Here's how the part is built. I have some questions about the finished solid (model axes, mm). A direction names the side the tool comes from. Round coordinates to 2 decimals unless told otherwise and drop trailing zeros. Loops run counter-clockwise (first coordinate to the right, second up) from the corner with the lowest first, then second, coordinate; pieces in that order, holes last. Notation, with made-up numbers: M 73,-15.5 L 107,-15.5 A25 ccw 107,10.5 Z; hole C -14,-2 d4. An arc over 180 degrees is marked long. Answer as CSV lines item,"result".
```python
from build123d import *

# Parameters (mm, degrees)
SKETCH1_R           = 6
SKETCH1_R_2         = 15
BOSS_EXTRUDE1_DEPTH = 5


with BuildPart() as part:
    # Sketch1 → Boss-Extrude1 (new body)
    with BuildSketch(Plane(origin=(0, 0, 0), x_dir=(1, 0, 0), z_dir=(0, 1, 0))):
        with BuildLine():
            Line((0, 0), (155, 0))
            Line((155, 0), (155, 20))
            ThreePointArc((155, 20), (152.071067812, 27.071067812), (145, 30))
            Line((145, 30), (119.160797831, 30))
            ThreePointArc((119.160797831, 30), (112.705825587, 32.362373842), (109.300664859, 38.333333333))
            ThreePointArc((109.300664859, 38.333333333), (95.355339059, 65.355339059), (68.333333333, 79.300664859))
            ThreePointArc((68.333333333, 79.300664859), (62.362373842, 82.705825587), (60, 89.160797831))
            Line((60, 89.160797831), (60, 100))
            ThreePointArc((60, 100), (57.071067812, 107.071067812), (50, 110))
            Line((50, 110), (10, 110))
            ThreePointArc((10, 110), (2.928932188, 107.071067812), (0, 100))
            Line((0, 100), (0, 0))
        make_face()
        with Locations((20, 15)):
            Circle(SKETCH1_R, mode=Mode.SUBTRACT)
        with Locations((40, 15)):
            Circle(SKETCH1_R, mode=Mode.SUBTRACT)
        with Locations((60, 15)):
            Circle(SKETCH1_R, mode=Mode.SUBTRACT)
        with Locations((80, 15)):
            Circle(SKETCH1_R, mode=Mode.SUBTRACT)
        with Locations((100, 15)):
            Circle(SKETCH1_R, mode=Mode.SUBTRACT)
        with Locations((120, 15)):
            Circle(SKETCH1_R, mode=Mode.SUBTRACT)
        with Locations((140, 15)):
            Circle(SKETCH1_R, mode=Mode.SUBTRACT)
        with Locations((30, 90)):
            Circle(SKETCH1_R_2, mode=Mode.SUBTRACT)
        with BuildLine():
            Line((60, 60), (30, 60))
            ThreePointArc((30, 60), (22.928932188, 57.071067812), (20, 50))
            Line((20, 50), (20, 40))
            ThreePointArc((20, 40), (22.928932188, 32.928932188), (30, 30))
            Line((30, 30), (77.320508076, 30))
            ThreePointArc((77.320508076, 30), (85.980762114, 35), (85.980762114, 45))
            ThreePointArc((85.980762114, 45), (75, 55.980762114), (60, 60))
        make_face(mode=Mode.SUBTRACT)
    extrude(amount=BOSS_EXTRUDE1_DEPTH)


solid = part.part
```
1. We'd pull the mould along X, two halves only. Please class faces 1 (the cylindrical face through (112.78, 2.46, -32.3)), 2 (the flat face through (76, 0, -56)), 3 (the cylindrical face through (22.85, 2.46, -33.01)): pulls with the +X half, pulls with the -X half, needs draft (parallel to the pull), parting line crosses it, or undercut.
Evaluation:
face 1,"pulls with the +X half"
face 2,"needs draft"
face 3,"undercut"
2. I want a section at A-A, the plane z = -15. Count the separate pieces of the cut face and the enclosed holes in it, and give its area (3 significant figures).
Evaluation:
separate pieces,"8"
enclosed holes,"0"
area,"355 mm²"
3. I want a section at B-B, the plane x = 140. Please give me the cut outline in (y, z), and give its area (3 significant figures).
Evaluation:
outline,"M 0,-30 L 5,-30 L 5,-21 L 0,-21 Z; M 0,-9 L 5,-9 L 5,0 L 0,0 Z"
area,"90.0 mm²"
4. Which directions (+Z, -Z, +X, -X, +Y, -Y) give clear straight access to the entire face, cutting with the end or side of a thin tool? Please do faces 4 (the cylindrical face through (75.19, 2.46, -55.87)), 5 (the flat face through (0, 2, -51)), 6 (the flat face through (132, 2, -30)).
Evaluation:
face 4,"+Y, -Y"
face 5,"+Z, -Z, -X, +Y, -Y"
face 6,"-Z, +X, +Y, -Y"
5. I want a section at D-D, the plane x = 40. Please give me the cut outline in (y, z), and give its area (3 significant figures).
Evaluation:
outline,"M 0,-110 L 5,-110 L 5,-101.18 L 0,-101.18 Z; M 0,-78.82 L 5,-78.82 L 5,-60 L 0,-60 Z; M 0,-30 L 5,-30 L 5,-21 L 0,-21 Z; M 0,-9 L 5,-9 L 5,0 L 0,0 Z"
area,"228 mm²"
6. If I drill on line 1 (Z direction, x = 30, y = 3.5); line 2 (Z direction, x = 140, y = 1.55); line 3 (Z direction, x = 77, y = 2.1), over which ranges is the centre line in solid material (lowest first)? Write a range as [from, to].
Evaluation:
line 1,"z = [-110, -105], [-75, -60], [-30, 0]"
line 2,"z = [-30, -21], [-9, 0]"
line 3,"z = [-77.02, -54.72], [-30, -20.2], [-9.8, 0]"
7. For P1, Ø2, axis at y = 3, z = -22, coming from the +X side, with a flat end and sliding along its axis, tell me the tip position at first contact or that it passes through.
Evaluation:
P1,"stops at x = 154.95"
